from build123d import *

# Parameters (mm, degrees)
SKETCH1_R           = 52.5
BOSS_EXTRUDE1_DEPTH = 30
SKETCH2_R           = 50.175
SKETCH2_R_2         = 44.85
CUT_EXTRUDE1_DEPTH  = 7
SKETCH3_R           = 42.85
SKETCH3_R_2         = 30
CUT_EXTRUDE2_DEPTH  = 20
SKETCH6_R           = 27.5
CUT_EXTRUDE6_DEPTH  = 81.07808689
SKETCH9_R           = 1.65
CUT_EXTRUDE7_DEPTH  = 10
SKETCH10_R          = 3
CUT_EXTRUDE8_DEPTH  = 4
SKETCH12_W          = 130.559751652
SKETCH12_H          = 125.592804578
CUT_EXTRUDE9_DEPTH  = 5
SKETCH13_R          = 43.441303223
SKETCH13_R_2        = 30
CUT_EXTRUDE10_DEPTH = 0.3


with BuildPart() as part:
    # Sketch1 → Boss-Extrude1 (new body)
    with BuildSketch(Plane(origin=(0, 0, 0), x_dir=(1, 0, 0), z_dir=(0, 1, 0))):
        with Locations(Location((0, 0, 0), (0, 0, 270))):
            Circle(SKETCH1_R)
    extrude(amount=BOSS_EXTRUDE1_DEPTH)

    # Sketch2 → Cut-Extrude1 (cut)
    with BuildSketch(Plane(origin=(0, 30, 0), x_dir=(1, 0, 0), z_dir=(0, 1, 0))):
        with Locations(Location((0, 0, 0), (0, 0, 270))):
            Circle(SKETCH2_R)
        with Locations(Location((0, 0, 0), (0, 0, 270))):
            Circle(SKETCH2_R_2, mode=Mode.SUBTRACT)
    extrude(amount=-CUT_EXTRUDE1_DEPTH, mode=Mode.SUBTRACT)

    # Sketch3 → Cut-Extrude2 (cut)
    with BuildSketch(Plane(origin=(0, 30, 0), x_dir=(1, 0, 0), z_dir=(0, 1, 0))):
        with Locations(Location((0, 0, 0), (0, 0, 270))):
            Circle(SKETCH3_R)
        with Locations(Location((0, 0, 0), (0, 0, 270))):
            Circle(SKETCH3_R_2, mode=Mode.SUBTRACT)
    extrude(amount=-CUT_EXTRUDE2_DEPTH, mode=Mode.SUBTRACT)

    # Sketch6 → Cut-Extrude6 (cut, through all)
    with BuildSketch(Plane(origin=(0, 30, 0), x_dir=(1, 0, 0), z_dir=(0, 1, 0))):
        with Locations(Location((0, 0, 0), (0, 0, 270))):
            Circle(SKETCH6_R)
    extrude(amount=-CUT_EXTRUDE6_DEPTH, mode=Mode.SUBTRACT)

    # Sketch9 → Cut-Extrude7 (cut)
    with BuildSketch(Plane.XZ):
        with Locations(Location((-25.635, 25.635, 0), (0, 0, 270))):
            Circle(SKETCH9_R)
        with Locations(Location((25.635, 25.635, 0), (0, 0, 270))):
            Circle(SKETCH9_R)
        with Locations(Location((25.635, -25.635, 0), (0, 0, 270))):
            Circle(SKETCH9_R)
        with Locations(Location((-25.635, -25.635, 0), (0, 0, 270))):
            Circle(SKETCH9_R)
    extrude(amount=-CUT_EXTRUDE7_DEPTH, mode=Mode.SUBTRACT)

    # Sketch10 → Cut-Extrude8 (cut)
    with BuildSketch(Plane.XZ):
        with Locations(Location((-25.635, 25.635, 0), (0, 0, 270))):
            Circle(SKETCH10_R)
        with Locations(Location((25.635, 25.635, 0), (0, 0, 270))):
            Circle(SKETCH10_R)
        with Locations(Location((25.635, -25.635, 0), (0, 0, 270))):
            Circle(SKETCH10_R)
        with Locations(Location((-25.635, -25.635, 0), (0, 0, 270))):
            Circle(SKETCH10_R)
    extrude(amount=-CUT_EXTRUDE8_DEPTH, mode=Mode.SUBTRACT)

    # Sketch12 → Cut-Extrude9 (cut)
    with BuildSketch(Plane(origin=(0, 30, 0), x_dir=(1, 0, 0), z_dir=(0, 1, 0))):
        Rectangle(SKETCH12_W, SKETCH12_H)
    extrude(amount=-CUT_EXTRUDE9_DEPTH, mode=Mode.SUBTRACT)

    # Sketch13 → Cut-Extrude10 (cut)
    with BuildSketch(Plane(origin=(0, 10, 0), x_dir=(1, 0, 0), z_dir=(0, 1, 0))):
        with Locations(Location((-0.591303223, 0, 0), (0, 0, 270))):
            Circle(SKETCH13_R)
        with Locations(Location((0, 0, 0), (0, 0, 270))):
            Circle(SKETCH13_R_2, mode=Mode.SUBTRACT)
    extrude(amount=-CUT_EXTRUDE10_DEPTH, mode=Mode.SUBTRACT)


solid = part.part
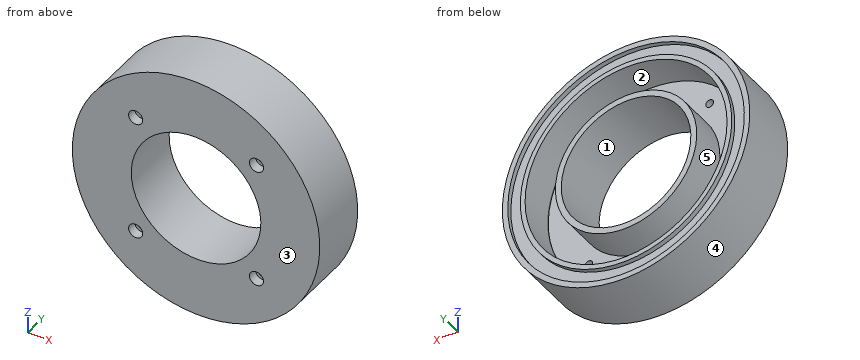
Work out the finished part from the listing and answer in its coordinate system (mm). Face numbers are marked on the shaded views. A direction names the side the tool comes from. Give positions to 0.01 mm unless a question says otherwise; leave off trailing zeros. Order: outer loops, then holes, each group sorted by start corner. A loop starts at its lowest first (then second) coordinate and runs counter-clockwise, first axis right, second up. Notation, with made-up numbers: (-33, -19.5) - (-18, -19.5) arc R13 cw to (-18, 1.5) - close; hole circle Ø10 at (-12.5, 87.25). An arc over 180 degrees is marked (long way). Answer as CSV lines item,"result". Start each with the question number.
Q1. The part is cut by section D-D (z = -34). Write down the section's boundary in (x, y).
Q2. Given pin 1 Ø4 at (y, z) = (22, 13.5) entering from +X (3 decimals); pin 2 Ø6 at (x, y) = (32, 3) entering from -Z; pin 3 Ø2.5 at (x, z) = (25.635, 25.635) entering from +Y; pin 4 Ø1.8 at (x, z) = (-26, 27) entering from -Y, each flat-ended and moving along its own axis, determine where each tip first touches the part or whether it passes through.
Q3. The part is cut by section C-C (x = 16). Write down the section's boundary in (y, z).
Q4. The mould has two halves that part along X. Classify the marked faces 3, 4 and 5: +X half, -X half, draft (parallel to the pull), parting line (faces both ways), or undercut.
Q5. Find the intervals of material crossed by L1, parallel to X at y = 11.25, z = 0; L2, parallel to X at y = 24.65, z = 0 (3 decimals); L3, parallel to X at y = 19.25, z = 12, in increasing order. Write a range as [from, to].
Q6. The part is cut by section A-A (y = 13). Write down the section's boundary in (x, z).
Q7. For the marked faces 1 and 2, determine the directions among +Z, -Z, +X, -X, +Y, -Y from which every point of the face is accessible in a straight line to the end or side of a thin tool.
Check result:
1,outline,"(-40, 0) - (40, 0) - (40, 25) - (36.9, 25) - (36.9, 23) - (29.25, 23) - (29.25, 25) - (26.08, 25) - (26.08, 10) - (26.45, 10) - (26.45, 9.7) - (-27.63, 9.7) - (-27.63, 10) - (-26.08, 10) - (-26.08, 25) - (-29.25, 25) - (-29.25, 23) - (-36.9, 23) - (-36.9, 25) - (-40, 25) - close"
2,pin 1,"stops at x = 51.225"
2,pin 2,"stops at z = -43.76"
2,pin 3,"passes through"
2,pin 4,"stops at y = 4"
3,outline,"(0, -50) - (25, -50) - (25, -47.56) - (23, -47.56) - (23, -41.9) - (25, -41.9) - (25, -39.75) - (10, -39.75) - (10, -40.15) - (9.7, -40.15) - (9.7, -25.38) - (25, -25.38) - (25, -22.37) - (0, -22.37) - close; (0, 22.37) - (25, 22.37) - (25, 25.38) - (9.7, 25.38) - (9.7, 40.15) - (10, 40.15) - (10, 39.75) - (25, 39.75) - (25, 41.9) - (23, 41.9) - (23, 47.56) - (25, 47.56) - (25, 50) - (0, 50) - close"
4,face 3,"draft"
4,face 4,"parting line"
4,face 5,"undercut"
5,L1,"x = [-52.5, -42.85], [-30, -27.5], [27.5, 30], [42.85, 52.5]"
5,L2,"x = [-52.5, -50.175], [-44.85, -42.85], [-30, -27.5], [27.5, 30], [42.85, 44.85], [50.175, 52.5]"
5,L3,"x = [-51.11, -41.14], [-27.5, -24.74], [24.74, 27.5], [41.14, 51.11]"
6,outline,"circle Ø105 at (0, 0); circle Ø60 at (0, 0); hole circle Ø85.7 at (0, 0); hole circle Ø55 at (0, 0)"
7,face 1,"+Y, -Y"
7,face 2,"+Y"
